from build123d import *

# Parameters (mm, degrees)
SKETCH_1_R          = 2.1
EXTRUDE_1_DEPTH     = 3
EXTRUDE_2_DEPTH     = 59
CUT_EXTRUDE_START   = -59
CUT_EXTRUDE_1_DEPTH = 59
CUT_EXTRUDE_2_DEPTH = 59
FILLET_3_DEPTH      = 3
SKETCH_7_W          = 4
SKETCH_7_H          = 59
EXTRUDE_3_DEPTH     = 15
SKETCH_8_R          = 2.75
CUT_EXTRUDE_3_DEPTH = 136
SKETCH_9_R          = 2.75
CUT_EXTRUDE_4_DEPTH = 136


with BuildPart() as part:
    # 草图1 → 凸台-拉伸1 (new body)
    with BuildSketch(Plane(origin=(0, 0, 0), x_dir=(1, 0, 0), z_dir=(0, 1, 0))):
        with BuildLine():
            ThreePointArc((-26.819805153, 31.819805153), (-30.355339059, 30.355339059), (-31.819805153, 26.819805153))
            Line((-31.819805153, 26.819805153), (-24, 19))
            Line((-24, 19), (-24, -19))
            Line((-24, -19), (-31.819805153, -26.819805153))
            ThreePointArc((-31.819805153, -26.819805153), (-30.355339059, -30.355339059), (-26.819805153, -31.819805153))
            Line((-26.819805153, -31.819805153), (-19, -24))
            Line((-19, -24), (19, -24))
            Line((19, -24), (26.819805153, -31.819805153))
            ThreePointArc((26.819805153, -31.819805153), (30.355339059, -30.355339059), (31.819805153, -26.819805153))
            Line((31.819805153, -26.819805153), (24, -19))
            Line((24, -19), (24, 19))
            Line((24, 19), (31.819805153, 26.819805153))
            ThreePointArc((31.819805153, 26.819805153), (30.355339059, 30.355339059), (26.819805153, 31.819805153))
            Line((26.819805153, 31.819805153), (19, 24))
            Line((19, 24), (-19, 24))
            Line((-19, 24), (-26.819805153, 31.819805153))
        make_face()
        with Locations(Location((-28.284271247, 28.284271247, 0), (0, 0, 270))):
            Circle(SKETCH_1_R, mode=Mode.SUBTRACT)
        with Locations(Location((-28.284271247, -28.284271247, 0), (0, 0, 270))):
            Circle(SKETCH_1_R, mode=Mode.SUBTRACT)
        with Locations(Location((28.284271247, 28.284271247, 0), (0, 0, 270))):
            Circle(SKETCH_1_R, mode=Mode.SUBTRACT)
        with Locations(Location((28.284271247, -28.284271247, 0), (0, 0, 270))):
            Circle(SKETCH_1_R, mode=Mode.SUBTRACT)
    extrude(amount=EXTRUDE_1_DEPTH)

    # 草图2 → 凸台-拉伸2 (add)
    with BuildSketch(Plane(origin=(0, 3, 0), x_dir=(1, 0, 0), z_dir=(0, 1, 0))):
        with BuildLine():
            Line((-11, -24), (-11, -19.5))
            Line((-11, -19.5), (-15.5, 0))
            ThreePointArc((-15.5, 0), (0, 15.5), (15.5, 0))
            Line((15.5, 0), (11, -19.5))
            Line((11, -19.5), (11, -24))
            Line((11, -24), (15, -24))
            Line((15, -24), (18.5, 0))
            ThreePointArc((18.5, 0), (0, 18.5), (-18.5, 0))
            Line((-18.5, 0), (-15, -24))
            Line((-15, -24), (-11, -24))
        make_face()
    extrude(amount=EXTRUDE_2_DEPTH)

    # 草图5 → 切除-拉伸1 (cut)
    with BuildSketch(Plane(origin=(0, 3, 0), x_dir=(1, 0, 0), z_dir=(0, 1, 0)).offset(CUT_EXTRUDE_START)):
        with BuildLine():
            Line((-15.5, 0), (-11, -19.5))
            Line((-11, -19.5), (-11, -24))
            Line((-11, -24), (11, -24))
            Line((11, -24), (11, -19.5))
            Line((11, -19.5), (15.5, 0))
            ThreePointArc((15.5, 0), (0, 15.5), (-15.5, 0))
        make_face()
    extrude(amount=CUT_EXTRUDE_1_DEPTH, mode=Mode.SUBTRACT)

    # 草图6 → 切除-拉伸2 (cut)
    with BuildSketch(Plane(origin=(0, 3, 0), x_dir=(1, 0, 0), z_dir=(0, 1, 0)).offset(CUT_EXTRUDE_START)):
        with BuildLine():
            Line((-15.340366038, 10.340366038), (-24, 19))
            Line((-24, 19), (-24, -19))
            Line((-24, -19), (-16.781818182, -11.781818182))
            Line((-16.781818182, -11.781818182), (-18.5, 0))
            ThreePointArc((-18.5, 0), (-17.692466924, 5.406164458), (-15.340366038, 10.340366038))
        make_face()
        with BuildLine():
            Line((-19, 24), (-10.629360281, 15.141555403))
            ThreePointArc((-10.629360281, 15.141555403), (-0.040504877, 18.499955658), (10.562955089, 15.187955089))
            Line((10.562955089, 15.187955089), (19, 24))
            Line((19, 24), (-19, 24))
        make_face()
        Polygon((-15, -24), (-15.509090909, -20.509090909), (-19, -24), align=None)
        with BuildLine():
            Line((24, 19), (15.141555403, 10.629360281))
            ThreePointArc((15.141555403, 10.629360281), (17.640419141, 5.573653427), (18.5, 0))
            Line((18.5, 0), (16.702005947, -12.329102079))
            Line((16.702005947, -12.329102079), (24, -19))
            Line((24, -19), (24, 19))
        make_face()
        Polygon((19, -24), (15.486287413, -20.665457737), (15, -24), align=None)
    extrude(amount=CUT_EXTRUDE_2_DEPTH, mode=Mode.SUBTRACT)

    # 圆角3: read off the stored shape, not the designer's step
    # 圆角3 outline → 圆角3 (add)
    with BuildSketch(Plane(origin=(0, 0, 0), x_dir=(1, 0, 0), z_dir=(0, 1, 0))):
        with BuildLine():
            Line((-16.781818182, -11.781818182), (-18.5, 0))
            ThreePointArc((-18.5, 0), (-19.698206739, -11.144620168), (-25.645540243, -20.645540243))
            Line((-25.645540243, -20.645540243), (-16.781818182, -11.781818182))
        make_face()
        with BuildLine():
            Line((19, -24), (15.486287413, -20.665457737))
            Line((15.486287413, -20.665457737), (15, -24))
            ThreePointArc((15, -24), (20.455899997, -26.47045686), (25.167660505, -30.167660505))
            Line((25.167660505, -30.167660505), (19, -24))
        make_face()
        with BuildLine():
            ThreePointArc((25.645540243, -20.645540243), (19.698206739, -11.144620168), (18.5, 0))
            Line((18.5, 0), (16.702005947, -12.329102079))
            Line((16.702005947, -12.329102079), (24, -19))
            Line((24, -19), (25.645540243, -20.645540243))
        make_face()
        with BuildLine():
            Line((24, 19), (15.141555403, 10.629360281))
            ThreePointArc((15.141555403, 10.629360281), (17.434869544, 6.186705422), (18.454815599, 1.292200137))
            ThreePointArc((18.454815599, 1.292200137), (19.976546369, 11.792519114), (25.716086069, 20.716086069))
            Line((25.716086069, 20.716086069), (24, 19))
        make_face()
        with BuildLine():
            ThreePointArc((20.716086069, 25.716086069), (11.792519114, 19.976546369), (1.292200137, 18.454815599))
            ThreePointArc((1.292200137, 18.454815599), (6.148517769, 17.448373255), (10.562955089, 15.187955089))
            Line((10.562955089, 15.187955089), (19, 24))
            Line((19, 24), (20.716086069, 25.716086069))
        make_face()
        with BuildLine():
            Line((-19, 24), (-10.629360281, 15.141555403))
            ThreePointArc((-10.629360281, 15.141555403), (-6.186705422, 17.434869544), (-1.292200137, 18.454815599))
            ThreePointArc((-1.292200137, 18.454815599), (-11.792519114, 19.976546369), (-20.716086069, 25.716086069))
            Line((-20.716086069, 25.716086069), (-19, 24))
        make_face()
        with BuildLine():
            ThreePointArc((-25.716086069, 20.716086069), (-19.976546369, 11.792519114), (-18.454815599, 1.292200137))
            ThreePointArc((-18.454815599, 1.292200137), (-17.492738551, 6.021137598), (-15.340366038, 10.340366038))
            Line((-15.340366038, 10.340366038), (-25.716086069, 20.716086069))
        make_face()
        with BuildLine():
            Line((-15, -24), (-15.509090909, -20.509090909))
            Line((-15.509090909, -20.509090909), (-25.167660505, -30.167660505))
            ThreePointArc((-25.167660505, -30.167660505), (-20.455899997, -26.47045686), (-15, -24))
        make_face()
    extrude(amount=FILLET_3_DEPTH)

    # 草图7 → 凸台-拉伸3 (add)
    with BuildSketch(Plane.XY.offset(24)):
        with Locations((-13, 32.5)):
            Rectangle(SKETCH_7_W, SKETCH_7_H)
        with Locations((13, 32.5)):
            Rectangle(SKETCH_7_W, SKETCH_7_H)
    extrude(amount=EXTRUDE_3_DEPTH)

    # 草图8 → 切除-拉伸3 (cut)
    with BuildSketch(Plane.XY):
        with Locations((0, 37)):
            Circle(SKETCH_8_R)
    extrude(amount=-CUT_EXTRUDE_3_DEPTH, mode=Mode.SUBTRACT)

    # 草图9 → 切除-拉伸4 (cut)
    with BuildSketch(Plane.ZY.offset(15)):
        with Locations((31.5, 42)):
            Circle(SKETCH_9_R)
        with Locations((31.5, 22)):
            Circle(SKETCH_9_R)
    extrude(amount=-CUT_EXTRUDE_4_DEPTH, mode=Mode.SUBTRACT)


solid = part.part
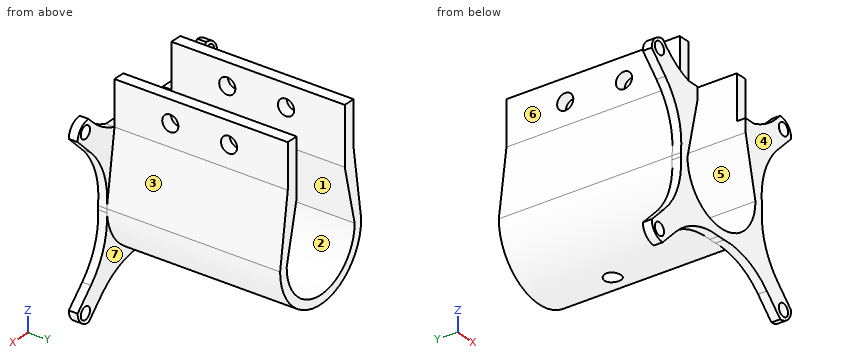
Design review of the part built by this model. Coordinates are the model's own, in mm. Face numbers are marked on the shaded views. A direction names the side the tool comes from. Coordinates: 2 decimals unless noted, no trailing zeros. Order: outer loops, then holes, each group sorted by start corner. A loop starts at its lowest first (then second) coordinate and runs counter-clockwise, first axis right, second up.
Item 1: Take a section at D-D, the plane y = 15.5. Write out the cut boundary in (x, z).
Item 2: For the marked faces 5, 6 and 7, list the 3-axis set-ups (+Z, -Z, +X, -X, +Y, -Y) from which the entire face can be reached by the end or side of a thin tool; tool diameter is ignored.
Item 3: Take a section at A-A, the plane y = 42. Write out the cut boundary in (x, z).
Item 4: For line 1 (X direction, y = 56, z = -0.5); line 2 (Y direction, x = -14, z = 31); line 3 (Y direction, x = 0, z = -16), list the stretches that pass through material, from the lowest coordinate up.
Item 5: For pin 1 Ø16.5 at (y, z) = (38.5, 34) entering from -X; pin 2 Ø5 at (y, z) = (30, -6) entering from +X; pin 3 Ø1 at (y, z) = (47.5, -2) entering from -X; pin 4 Ø4.5 at (x, y) = (0, 37) entering from -Z, all flat-tipped, find the tip position at first contact; note any pin that passes through.
Item 6: Take a section at C-C, the plane z = -9. Write out the cut boundary in (x, y).
Item 7: Take a section at B-B, the plane x = 0. Write out the cut boundary in (y, z).
Item 8: The part is to be moulded in two halves that separate along Z. For the marked faces 1, 2, 3 and 4, say which applies: pulls with the +Z half, pulls with the -Z half, needs draft (parallel to the pull), parting line crosses it, or undercut.
The answers:
1. outline: (-18.5, 0) arc R18.5 ccw to (18.5, 0) - (15, 24) - (15, 39) - (11, 39) - (11, 19.5) - (15.5, 0) arc R15.5 cw to (-15.5, 0) - (-11, 19.5) - (-11, 39) - (-15, 39) - (-15, 24) - close
2. face 5: +Y, -Y
2. face 6: +Z, -X, +Y, -Y
2. face 7: -Z, +X, +Y
3. outline: (-18.5, 0) arc R18.5 ccw to (18.5, 0) - (15, 24) - (15, 28.75) - (11, 28.75) - (11, 19.5) - (15.5, 0) arc R15.5 cw to (-15.5, 0) - (-11, 19.5) - (-11, 28.75) - (-15, 28.75) - (-15, 24) - close; (-15, 34.25) - (-11, 34.25) - (-11, 39) - (-15, 39) - close; (11, 34.25) - (15, 34.25) - (15, 39) - (11, 39) - close
4. line 1: x = -18.49 to -15.49, 15.49 to 18.49
4. line 2: y = 3 to 19.3, 24.7 to 39.3, 44.7 to 62
4. line 3: y = 0 to 34.25, 39.75 to 62
5. pin 1: stops at x = -15
5. pin 2: stops at x = 18.17
5. pin 3: stops at x = -18.44
5. pin 4: passes through
6. outline: (-19.11, 0) - (-12.62, 0) - (-12.62, 62) - (-16.16, 62) - (-16.16, 3) - (-19.11, 3) - close; (12.62, 0) - (19.11, 0) - (19.11, 3) - (16.16, 3) - (16.16, 62) - (12.62, 62) - close
7. outline: (0, -18.5) - (34.25, -18.5) - (34.25, -15.5) - (0, -15.5) - close; (39.75, -18.5) - (62, -18.5) - (62, -15.5) - (39.75, -15.5) - close
8. face 1: undercut
8. face 2: undercut
8. face 3: pulls with the +Z half
8. face 4: needs draft
